Geometry: final body of the model. Coordinates: model frame, mm. Give positions to 0.01 mm unless a question says otherwise; leave off trailing zeros. Write each loop counter-clockwise with the first axis right and the second up, starting at its lowest first coordinate (ties: lowest second). Pieces come first, ordered by that corner, then holes. Notation, with made-up numbers: (21, 49.5) - (38, 49.5) arc R20 cw to (38, 88.5) - close; hole circle Ø9 at (49, -5.5). An arc over 180 degrees is marked (long way). One line per question, with ' | ' between items. Start each with the question number.
```python
from build123d import *

# Parameters (mm, degrees)
F0_W     = 8.295227
F0_H     = 38.326367
F1_DEPTH = 27.662443
F2_R     = 5.08
F3_R     = 2.121776
F4_DEPTH = 25.4


with BuildPart() as f1:
    # F0 (on Top) → F1 (new body)
    with BuildSketch(Plane.XY):
        with Locations((-51.453689, -5.27262)):
            Rectangle(F0_W, F0_H)
    extrude(amount=F1_DEPTH)

    # F2
    f2_edges = [f1.edges().sort_by_distance(p)[0] for p in [
        (-51.453689, -24.435803, 27.662443),
    ]]
    fillet(f2_edges, radius=F2_R)

    # F3 (on face) → F4 (cut)
    with BuildSketch(Plane(origin=(-55.601303, 0, 0), x_dir=(0, -1, 0), z_dir=(-1, 0, 0))):
        with Locations((20.858478, 24.050102)):
            Circle(F3_R)
    extrude(amount=-F4_DEPTH, mode=Mode.SUBTRACT)


solid = f1.part
```
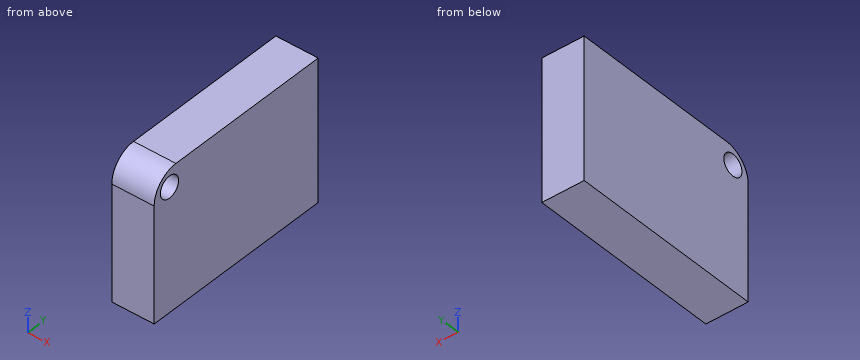
1) Line query: L1, parallel to Z at x = -53.5, y = -19; L2, parallel to Y at x = -54.5, z = 24.75. Output: solid intervals per line, ascending.
2) Section B-B, the plane y = -20. Output: boundary loops of the cut face in (x, z).
3) Section C-C, the plane x = -53.25. Output: boundary loops of the cut face in (y, z), plus the area to 3 significant figures.
4) Section A-A, the plane z = 23.5. Output: boundary loops of the cut face in (x, y).
Answer key:
1) L1: 0 to 23.03, 25.07 to 27.66 | L2: -23.95 to -22.86, -18.86 to 13.89
2) outline: (-55.6, 0) - (-47.31, 0) - (-47.31, 22.11) - (-55.6, 22.11) - close; (-55.6, 25.99) - (-47.31, 25.99) - (-47.31, 27.62) - (-55.6, 27.62) - close
3) outline: (-24.44, 0) - (13.89, 0) - (13.89, 27.66) - (-19.36, 27.66) arc R5.08 ccw to (-24.44, 22.58) - close; hole circle Ø4.24 at (-20.86, 24.05) | area: 1,040 mm^2
4) outline: (-55.6, -24.35) - (-47.31, -24.35) - (-47.31, -22.91) - (-55.6, -22.91) - close; (-55.6, -18.81) - (-47.31, -18.81) - (-47.31, 13.89) - (-55.6, 13.89) - close
